```python
from build123d import *

# Parameters (mm, degrees)
SKETCH1_R           = 1.8
SKETCH1_R_2         = 1.5
SKETCH1_W           = 7.5
SKETCH1_H           = 60
BOSS_EXTRUDE1_DEPTH = 5.08


with BuildPart() as part:
    # Sketch1 → Boss-Extrude1 (new body)
    with BuildSketch(Plane(origin=(0, 0, 0), x_dir=(0, 1, 0), z_dir=(0, 0, 1))):
        Polygon((-41.181536726, 53.881536726), (-19.05, 53.881536726), (-12.7, 60.231536726), (12.7, 60.231536726), (19.05, 53.881536726), (41.181536726, 53.881536726), (53.881536726, 41.181536726), (53.881536726, -41.181536726), (41.181536726, -53.881536726), (19.05, -53.881536726), (12.7, -60.231536726), (-12.7, -60.231536726), (-19.05, -53.881536726), (-41.181536726, -53.881536726), (-53.881536726, -41.181536726), (-53.881536726, 41.181536726), align=None)
        with Locations((-46.633511114, -37.653254993)):
            Circle(SKETCH1_R, mode=Mode.SUBTRACT)
        with Locations((-37.653254993, -46.633511114)):
            Circle(SKETCH1_R, mode=Mode.SUBTRACT)
        with Locations((46.633511114, -37.653254993)):
            Circle(SKETCH1_R, mode=Mode.SUBTRACT)
        with Locations((37.653254993, -46.633511114)):
            Circle(SKETCH1_R, mode=Mode.SUBTRACT)
        with Locations((-46.633511114, 37.653254993)):
            Circle(SKETCH1_R, mode=Mode.SUBTRACT)
        with Locations((-37.653254993, 46.633511114)):
            Circle(SKETCH1_R, mode=Mode.SUBTRACT)
        with Locations((37.653254993, 46.633511114)):
            Circle(SKETCH1_R, mode=Mode.SUBTRACT)
        with Locations((46.633511114, 37.653254993)):
            Circle(SKETCH1_R, mode=Mode.SUBTRACT)
        with Locations((-23, 43)):
            Circle(SKETCH1_R_2, mode=Mode.SUBTRACT)
        with Locations((23, 43)):
            Circle(SKETCH1_R_2, mode=Mode.SUBTRACT)
        with Locations((-23, -43)):
            Circle(SKETCH1_R_2, mode=Mode.SUBTRACT)
        with Locations((23, -43)):
            Circle(SKETCH1_R_2, mode=Mode.SUBTRACT)
        with Locations((9.525, -56.421536726)):
            Circle(SKETCH1_R, mode=Mode.SUBTRACT)
        with Locations((-9.525, -56.421536726)):
            Circle(SKETCH1_R, mode=Mode.SUBTRACT)
        with Locations((-9.525, 56.421536726)):
            Circle(SKETCH1_R, mode=Mode.SUBTRACT)
        with Locations((9.525, 56.421536726)):
            Circle(SKETCH1_R, mode=Mode.SUBTRACT)
        with Locations((-36, 0)):
            Rectangle(SKETCH1_W, SKETCH1_H, mode=Mode.SUBTRACT)
        with Locations((36, 0)):
            Rectangle(SKETCH1_W, SKETCH1_H, mode=Mode.SUBTRACT)
    extrude(amount=BOSS_EXTRUDE1_DEPTH)


solid = part.part
```
Geometry check sheet. Reference: the model listing, model coordinates, mm. A direction names the side the tool comes from. Coordinates: 2 decimals unless noted, no trailing zeros. Loops run counter-clockwise (first coordinate to the right, second up) from the corner with the lowest first, then second, coordinate; pieces in that order, holes last. Notation, with made-up numbers: (-7.75, -2) - (17.25, -2) arc R18 ccw to (17.25, 14) - close; hole circle Ø11 at (6, -3). An arc over 180 degrees is marked (long way). One line per item, written item: value. Start each with the question number.
(1) Material ranges on line 1 (Y direction, x = 29.5, z = 2.15); line 2 (Y direction, x = -47, z = 2.5); line 3 (X direction, y = 8, z = 2.25), recorded low to high. Write a range as [from, to].
(2) Tool access check on faces 1 (the flat face through (-53.882, 30, 3)), 2 (the flat face through (0, 39.75, 3)), 3 (the flat face through (53.882, 30, 3)). Record the directions out of +Z, -Z, +X, -X, +Y, -Y that give a thin tool (end or side, any length) a straight path to the whole face; none if there is none.
(3) Cross-section at B-B on x = 2. Enter the section's corners in (y, z).
(4) Cross-section at A-A on y = -23. Enter the section's corners in (x, z), plus the area to 3 significant figures.
(5) Cross-section at C-C on z = 1.3. Count the separate pieces of the cut face and the enclosed holes in it, plus the area to 3 significant figures.
(6) Mould release check, pull along X, two halves, no side actions. Record for faces 4 (the flat face through (30, -36, 3)), 5 (the flat face through (-1, 1, 0)), 6 (the flat face through (-60.232, 0, 3)): released by +X, released by -X, zero draft, split by the parting line, or undercut.
(7) Depth check by flat-ended pin: P1, Ø2, axis at x = -26.5, y = 23.5, coming from the -Z side; P2, Ø3, axis at y = 26, z = 4, coming from the +X side; P3, Ø3, axis at x = 46.63, y = -37.65, coming from the +Z side; P4, Ø1.5, axis at y = -34.5, z = 3, coming from the -X side. Enter the tip coordinate at first touch or a pass-through.
Results below:
1. line 1: y = [-53.88, -39.75], [-32.25, 32.25], [39.75, 53.88]
1. line 2: y = [-48.06, -39.42], [-35.89, 35.89], [39.42, 48.06]
1. line 3: x = [-60.23, -57.38], [-55.47, 55.47], [57.38, 60.23]
2. face 1: +Z, -Z, -X, +Y
2. face 2: +Z, -Z
2. face 3: +Z, -Z, +X, +Y
3. outline: (-53.88, 0) - (-39.75, 0) - (-39.75, 5.08) - (-53.88, 5.08) - close; (-32.25, 0) - (32.25, 0) - (32.25, 5.08) - (-32.25, 5.08) - close; (39.75, 0) - (53.88, 0) - (53.88, 5.08) - (39.75, 5.08) - close
4. outline: (-53.88, 0) - (-44.5, 0) - (-44.5, 5.08) - (-53.88, 5.08) - close; (-41.5, 0) - (41.5, 0) - (41.5, 5.08) - (-41.5, 5.08) - close; (44.5, 0) - (53.88, 0) - (53.88, 5.08) - (44.5, 5.08) - close
4. area: 517 mm2
5. separate pieces: 1
5. enclosed holes: 18
5. area: 10,600 mm2
6. face 4: undercut
6. face 5: zero draft
6. face 6: released by -X
7. P1: stops at z = 0
7. P2: stops at x = 53.88
7. P3: passes through
7. P4: stops at x = -53.88
